from build123d import *

# Parameters (mm, degrees)
F3_DEPTH = 2.54
F4_DEPTH = 1.27


with BuildPart() as f1:
    # F0 (on Front) → F1 (revolve)
    with BuildSketch(Plane.XZ):
        with BuildLine():
            Line((-10.16, 0), (0, 0))
            Line((0, 0), (0, 38.1))
            Line((0, 38.1), (-10.16, 38.1))
            Line((-10.16, 38.1), (-10.16, 35.56))
            ThreePointArc((-10.16, 35.56), (-6.8363821432, 34.5835975271), (-5.3975, 31.4325))
            ThreePointArc((-5.3975, 31.4325), (-4.5044566757, 21.6875293186), (-4.206875, 11.90625))
            Line((-4.206875, 11.90625), (-4.60375, 11.90625))
            Line((-4.60375, 11.90625), (-4.60375, 11.1125))
            Line((-4.60375, 11.1125), (-5.3975, 11.1125))
            Line((-5.3975, 11.1125), (-5.3975, 9.525))
            Line((-5.3975, 9.525), (-6.985, 9.525))
            Line((-6.985, 9.525), (-6.985, 6.35))
            Line((-6.985, 6.35), (-10.16, 6.35))
            Line((-10.16, 6.35), (-10.16, 0))
        make_face()
    revolve(axis=Axis((0, 0, 19.05), (0, 0, -1)))

    # F2 (on face) → F3 (cut)
    with BuildSketch(Plane.XY.offset(38.1)):
        with BuildLine():
            ThreePointArc((0.635, -7.5934955719), (5.3881536726, -5.3881536726), (7.5934955719, -0.635))
            Line((7.5934955719, -0.635), (0.635, -0.635))
            Line((0.635, -0.635), (0.635, -7.5934955719))
        make_face()
        with BuildLine():
            ThreePointArc((-0.635, -7.5934955719), (0, -7.62), (0.635, -7.5934955719))
            Line((0.635, -7.5934955719), (0.635, -0.635))
            Line((0.635, -0.635), (0, -0.635))
            Line((0, -0.635), (-0.635, -0.635))
            Line((-0.635, -0.635), (-0.635, -7.5934955719))
        make_face()
        with BuildLine():
            ThreePointArc((-7.5934955719, -0.635), (-5.3881536726, -5.3881536726), (-0.635, -7.5934955719))
            Line((-0.635, -7.5934955719), (-0.635, -0.635))
            Line((-0.635, -0.635), (-7.5934955719, -0.635))
        make_face()
        with BuildLine():
            Line((-0.635, 0.635), (-7.5934955719, 0.635))
            ThreePointArc((-7.5934955719, 0.635), (-7.62, 0), (-7.5934955719, -0.635))
            Line((-7.5934955719, -0.635), (-0.635, -0.635))
            Line((-0.635, -0.635), (-0.635, 0))
            Line((-0.635, 0), (-0.635, 0.635))
        make_face()
        with BuildLine():
            Line((-0.635, 0.635), (-0.635, 7.5934955719))
            ThreePointArc((-0.635, 7.5934955719), (-5.3881536726, 5.3881536726), (-7.5934955719, 0.635))
            Line((-7.5934955719, 0.635), (-0.635, 0.635))
        make_face()
        with BuildLine():
            Line((0.635, 0.635), (0.635, 7.5934955719))
            ThreePointArc((0.635, 7.5934955719), (0, 7.62), (-0.635, 7.5934955719))
            Line((-0.635, 7.5934955719), (-0.635, 0.635))
            Line((-0.635, 0.635), (0, 0.635))
            Line((0, 0.635), (0.635, 0.635))
        make_face()
        with BuildLine():
            Line((0.635, 0.635), (7.5934955719, 0.635))
            ThreePointArc((7.5934955719, 0.635), (5.3881536726, 5.3881536726), (0.635, 7.5934955719))
            Line((0.635, 7.5934955719), (0.635, 0.635))
        make_face()
        Polygon((0.635, 0), (0.635, 0.635), (0, 0.635), (-0.635, 0.635), (-0.635, 0), (-0.635, -0.635), (0, -0.635), (0.635, -0.635), align=None)
        with BuildLine():
            ThreePointArc((7.5934955719, -0.635), (7.6133710095, -0.3177764484), (7.62, 0))
            ThreePointArc((7.62, 0), (7.6133710095, 0.3177764484), (7.5934955719, 0.635))
            Line((7.5934955719, 0.635), (0.635, 0.635))
            Line((0.635, 0.635), (0.635, 0))
            Line((0.635, 0), (0.635, -0.635))
            Line((0.635, -0.635), (7.5934955719, -0.635))
        make_face()
    extrude(amount=-F3_DEPTH, mode=Mode.SUBTRACT)

    # F2 (on face) → F4 (cut)
    with BuildSketch(Plane.XY.offset(38.1)):
        with BuildLine():
            ThreePointArc((-7.5934955719, -0.635), (-7.62, 0), (-7.5934955719, 0.635))
            Line((-7.5934955719, 0.635), (-10.1401368334, 0.635))
            ThreePointArc((-10.1401368334, 0.635), (-10.1550329942, 0.3176552949), (-10.16, 0))
            ThreePointArc((-10.16, 0), (-10.1550329942, -0.3176552949), (-10.1401368334, -0.635))
            Line((-10.1401368334, -0.635), (-7.5934955719, -0.635))
        make_face()
        with BuildLine():
            ThreePointArc((-0.635, 7.5934955719), (0, 7.62), (0.635, 7.5934955719))
            Line((0.635, 7.5934955719), (0.635, 10.1401368334))
            ThreePointArc((0.635, 10.1401368334), (0.3176552949, 10.1550329942), (0, 10.16))
            ThreePointArc((0, 10.16), (-0.3176552949, 10.1550329942), (-0.635, 10.1401368334))
            Line((-0.635, 10.1401368334), (-0.635, 7.5934955719))
        make_face()
        with BuildLine():
            ThreePointArc((7.5934955719, 0.635), (7.6133710095, 0.3177764484), (7.62, 0))
            ThreePointArc((7.62, 0), (7.6133710095, -0.3177764484), (7.5934955719, -0.635))
            Line((7.5934955719, -0.635), (10.1401368334, -0.635))
            ThreePointArc((10.1401368334, -0.635), (10.1550329942, -0.3176552949), (10.16, 0))
            ThreePointArc((10.16, 0), (10.1550329942, 0.3176552949), (10.1401368334, 0.635))
            Line((10.1401368334, 0.635), (7.5934955719, 0.635))
        make_face()
        with BuildLine():
            Line((0.635, -10.1401368334), (0.635, -7.5934955719))
            ThreePointArc((0.635, -7.5934955719), (0, -7.62), (-0.635, -7.5934955719))
            Line((-0.635, -7.5934955719), (-0.635, -10.1401368334))
            ThreePointArc((-0.635, -10.1401368334), (-0.3176552949, -10.1550329942), (0, -10.16))
            ThreePointArc((0, -10.16), (0.3176552949, -10.1550329942), (0.635, -10.1401368334))
        make_face()
    extrude(amount=-F4_DEPTH, mode=Mode.SUBTRACT)


solid = f1.part
Input: part model. Units: mm. Frame: model coordinates. A direction names the side the tool comes from. Give positions to 0.01 mm unless a question says otherwise; leave off trailing zeros. Loops run counter-clockwise (first coordinate to the right, second up) from the corner with the lowest first, then second, coordinate; pieces in that order, holes last. Notation, with made-up numbers: M -25.5,61 L 20.5,61 A24 cw 20.5,92 Z; hole C 31.5,43 d5. An arc over 180 degrees is marked long. Use one line per item in the form item = value.
1. Pull-direction query (Y, two-part tool) for faces 1 (the face through (3.653, -2.801, 11.504)), 2 (the face through (-9, 0.635, 37)), 3 (the face through (6, -5, 38.1)); classes: released by +Y, released by -Y, zero draft, split by the parting line, or undercut.
Numbers:
face_1 = split by the parting line
face_2 = undercut
face_3 = zero draft
2. Section query C-C, the plane z = 25. Return the cut outline in (x, y).
Numbers:
outline = C 0,0 d9.48
3. First-contact query: pin 1 (1 mm diameter, centred on x = -9.5, z = 37.5, fed in from +Y); pin 2 (8 mm diameter, centred on y = -0.5, z = 25.5, fed in from -X); pin 3 (0.6 mm diameter, centred on x = 9, y = 0, fed in from +Z); pin 4 (1 mm diameter, centred on x = -6.5, y = -5.5, fed in from -Z). Flat tips, straight axial feed; report the tip coordinate or a pass-through.
Numbers:
pin_1 = 4.71
pin_2 = -5.17
pin_3 = 36.83
pin_4 = 0
4. Reachability of faces 4 (the face through (4, -4, 9.525)), 5 (the face through (0, 0, 35.56)), 6 (the face through (9, 0.635, 37)), 7 (the face through (0.635, -9, 37)) from +Z, -Z, +X, -X, +Y, -Y: full face, straight path, thin tool, end or side. Return the list, or none.
Numbers:
face_4 = none
face_5 = +Z
face_6 = +Z, +X, -X
face_7 = +Z, +Y, -Y
5. Line query: L1, parallel to Z at x = 6.5, y = -7.75; L2, parallel to Y at x = -0.5, z = 4; L3, parallel to Z at x = 4.5, y = 4.75 (3 decimals). Output: solid intervals per line, ascending.
Numbers:
L1 = 0 to 6.35, 35.57 to 38.1
L2 = -10.15 to 10.15
L3 = 0 to 9.525, 34.303 to 35.56
6. Section query B-B, the plane z = 16. Return the cut outline in (x, y).
Numbers:
outline = C 0,0 d8.52
